```python
from build123d import *

# Parameters (mm, degrees)
SKETCH_1_R      = 1.65
EXTRUDE_1_DEPTH = 5
CHAMFER_1_SIZE  = 0.6


with BuildPart() as part:
    # 草图1 → 凸台-拉伸1 (new body)
    with BuildSketch(Plane.XY):
        with BuildLine():
            Line((-36, 4), (36, 4))
            ThreePointArc((36, 4), (40, 0), (36, -4))
            Line((36, -4), (-36, -4))
            ThreePointArc((-36, -4), (-40, 0), (-36, 4))
        make_face()
        with Locations((-36, 0)):
            Circle(SKETCH_1_R, mode=Mode.SUBTRACT)
        with Locations((36, 0)):
            Circle(SKETCH_1_R, mode=Mode.SUBTRACT)
    extrude(amount=EXTRUDE_1_DEPTH)

    # 倒角1
    chamfer_1_edges = [part.edges().sort_by_distance(p)[0] for p in [
        (-37.65, 0, 0),
        (-37.65, 0, 5),
        (40, 0, 5),
        (34.35, 0, 0),
        (34.35, 0, 5),
        (0, 4, 5),
        (-40, 0, 5),
        (0, 4, 0),
        (40, 0, 0),
        (0, -4, 0),
        (-40, 0, 0),
        (0, -4, 5),
    ]]
    chamfer(chamfer_1_edges, length=CHAMFER_1_SIZE)


solid = part.part
```
Input: part model. Units: mm. Frame: model coordinates. Coordinates: 2 decimals unless noted, no trailing zeros. Loops run counter-clockwise (first coordinate to the right, second up) from the corner with the lowest first, then second, coordinate; pieces in that order, holes last. Notation, with made-up numbers: M 11.25,30 L 45.25,30 A31 ccw 45.25,56 Z; hole C 78.25,28 d1. An arc over 180 degrees is marked long. Answer in a Markdown table with one row per item.
1. Section A-A, the plane y = 0. Output: boundary loops of the cut face in (x, z).
Response:
| item | result |
|---|---|
| outline | M -40,0.6 L -39.4,0 L -38.25,0 L -37.65,0.6 L -37.65,4.4 L -38.25,5 L -39.4,5 L -40,4.4 Z; M -34.35,0.6 L -33.75,0 L 33.75,0 L 34.35,0.6 L 34.35,4.4 L 33.75,5 L -33.75,5 L -34.35,4.4 Z; M 37.65,0.6 L 38.25,0 L 39.4,0 L 40,0.6 L 40,4.4 L 39.4,5 L 38.25,5 L 37.65,4.4 Z |
2. Material intervals for line 1 (Y direction, x = 36, z = 2.15); line 2 (X direction, y = 1.25, z = 3.7); line 3 (X direction, y = 0.75, z = 3.9), sorted ascending.
Response:
| item | result |
|---|---|
| line 1 | y = -4 to -1.65, 1.65 to 4 |
| line 2 | x = -39.8 to -37.08, -34.92 to 34.92, 37.08 to 39.8 |
| line 3 | x = -39.93 to -37.47, -34.53 to 34.53, 37.47 to 39.93 |
3. Section C-C, the plane x = 19.5. Output: boundary loops of the cut face in (y, z), then the cut area to 3 significant figures.
Response:
| item | result |
|---|---|
| outline | M -4,0.6 L -3.4,0 L 3.4,0 L 4,0.6 L 4,4.4 L 3.4,5 L -3.4,5 L -4,4.4 Z |
| area | 39.3 mm2 |
4. Section B-B, the plane z = 3.25. Output: boundary loops of the cut face in (x, y), then the cut area to 3 significant figures.
Response:
| item | result |
|---|---|
| outline | M -36,-4 L 36,-4 A4 ccw 36,4 L -36,4 A4 ccw Z; hole C -36,0 d3.3; hole C 36,0 d3.3 |
| area | 609 mm2 |
5. Draft query along X for faces 1 (the conical face through (39.6, 0.1, 4.8)), 2 (the conical face through (-39.6, -0.1, 4.8)), 3 (the cylindrical face through (-37.65, 0.07, 2.47)). Return one class per face: pulls with the +X half, pulls with the -X half, needs draft (parallel to the pull), parting line crosses it, or undercut.
Response:
| item | result |
|---|---|
| face 1 | pulls with the +X half |
| face 2 | pulls with the -X half |
| face 3 | undercut |
6. First-contact query: pin 1 (2 mm diameter, centred on x = -36, y = 0, fed in from +Z); pin 2 (4 mm diameter, centred on x = 36, y = 0, fed in from -Z); pin 3 (2 mm diameter, centred on y = -2, z = 2, fed in from +X). Flat tips, straight axial feed; report the tip coordinate or a pass-through.
Response:
| item | result |
|---|---|
| pin 1 | passes through |
| pin 2 | stops at z = 0.25 |
| pin 3 | stops at x = 39.87 |
